Part model, mm, in its own coordinate system. A direction names the side the tool comes from. Round coordinates to 2 decimals unless told otherwise and drop trailing zeros. Write each loop counter-clockwise with the first axis right and the second up, starting at its lowest first coordinate (ties: lowest second). Pieces come first, ordered by that corner, then holes. Notation, with made-up numbers: (69, 18) -> (127, 18) arc R21 cw to (127, 26) -> close; hole circle Ø4 at (-9.5, 10.5). An arc over 180 degrees is marked (long way). Return JSON: item names as keys, results as strings. Group by question number.
```python
from build123d import *

# Parameters (mm, degrees)
F0_W     = 254
F0_H     = 203.2
F1_DEPTH = 193.04
F2_R     = 127
F3_SIZE  = 50.8
F4_T     = -25.4


with BuildPart() as f1:
    # F0 (on Front) → F1 (new body)
    with BuildSketch(Plane.XZ):
        with Locations((3.474914, 28.0605)):
            Rectangle(F0_W, F0_H)
    extrude(amount=F1_DEPTH)

    # F2
    f2_edges = [f1.edges().sort_by_distance(p)[0] for p in [
        (3.474914, -193.04, 129.6605),
    ]]
    fillet(f2_edges, radius=F2_R)

    # F3
    f3_edges = [f1.edges().sort_by_distance(p)[0] for p in [
        (3.474914, 0, -73.5395),
    ]]
    chamfer(f3_edges, length=F3_SIZE)

    # F4
    f4_openings = [f1.faces().sort_by_distance(p)[0] for p in [
        (130.474914, -92.656111, 23.8767),
    ]]
    offset(amount=F4_T, openings=f4_openings)


solid = f1.part
```
Item 1: Cut at C-C (z = -33.5). Write the cut outline in (x, y), then the cut area to 3 significant figures.
Item 2: Cut at B-B (y = -42.5). Write the cut outline in (x, z).
Item 3: Two-plate mould, pull along Z, no slides. Class faces 1 (the face through (5.253, -154.85, 93.445)), 2 (the face through (-123.525, -95, 27)), 3 (the face through (-98.125, -96, 27)): released by +Z, released by -Z, zero draft, split by the parting line, or undercut.
Item 4: Which spindle directions (+Z, -Z, +X, -X, +Y, -Y) get a long thin tool onto all of the face, cutting with end or side? Do faces 4 (the face through (15, -114, -48.139)), 5 (the face through (1.7, -25.76, -48.5)). Say none if no direction does.
Item 5: Wall check: L1, parallel to X at y = -131.5, z = 70.5; L2, parallel to Y at x = 34, z = 48.5; L3, parallel to Y at x = -87, z = -39.5. Give the ranges that are in metal, low to high.
Item 6: Cut at A-A (x = 38). Write the cut outline in (y, z), then the cut area to 3 significant figures.
Item 7: Flat gauge pins, fed straight in: P1, Ø15, axis at x = -20.5, z = -31.5, coming from the +Y side; P2, Ø1.5, axis at x = -98, z = 64.5, coming from the -Y side; P3, Ø12, axis at y = -127, z = -37.5, coming from the +X side. Where does each tip first touch, or does it go through?
Checks:
{
 "1": {"outline": "(-123.53, -193.04) -> (130.47, -193.04) -> (130.47, -167.64) -> (-98.13, -167.64) -> (-98.13, -46.68) -> (130.47, -46.68) -> (130.47, -10.76) -> (-123.53, -10.76) -> close", "area": "18,600 mm2"},
 "2": {"outline": "(-123.53, -65.24) -> (130.47, -65.24) -> (130.47, -29.32) -> (-98.13, -29.32) -> (-98.13, 104.26) -> (130.47, 104.26) -> (130.47, 129.66) -> (-123.53, 129.66) -> close"},
 "3": {"face 1": "released by +Z", "face 2": "zero draft", "face 3": "undercut"},
 "4": {"face 4": "+X", "face 5": "-Z, +X, -X, +Y"},
 "5": {"L1": "x = -123.53 to -98.13", "L2": "y = -184.48 to -156.71, -25.4 to 0", "L3": "y = -193.04 to -167.64, -52.68 to -16.76"},
 "6": {"outline": "(-193.04, -73.54) -> (-50.8, -73.54) -> (0, -22.74) -> (0, 129.66) -> (-66.04, 129.66) arc R127 ccw to (-193.04, 2.66) -> close; hole (-167.64, -48.14) -> (-61.32, -48.14) -> (-25.4, -12.22) -> (-25.4, 104.26) -> (-66.04, 104.26) arc R101.6 ccw to (-167.64, 2.66) -> close", "area": "15,700 mm2"},
 "7": {"P1": "stops at y = -1.26", "P2": "stops at y = -177.38", "P3": "stops at x = -98.13"}
}
